For this review, take the finished solid that the model builds, in its own axes (mm). A direction names the side the tool comes from. Give positions to 0.01 mm unless a question says otherwise; leave off trailing zeros. Order: outer loops, then holes, each group sorted by start corner. A loop starts at its lowest first (then second) coordinate and runs counter-clockwise, first axis right, second up. Notation, with made-up numbers: M -20,75 L -15,75 A21 cw -15,106 Z; hole C -3,58 d6. An arc over 180 degrees is marked long. Use CSV: the item, a comma, the result in double quotes. Start each with the question number.
(1) Consider section C-C (z = -24.5). Write out the cut boundary in (x, y).
(2) Tool access review of faces 1 (the face through (51, 825, -4)), 2 (the face through (49, 828, 0)): name each direction out of +Z, -Z, +X, -X, +Y, -Y from which nothing blocks a thin tool from reaching the whole face with its end or side.
(3) Draft analysis for pull direction Z (two halves, no side actions). For faces 3 (the face through (97.915, 119.104, -46.063)), 4 (the face through (46, 1500, -2)), 5 (the face through (96, 771, -51)), state which applies: pulls with the +Z half, pulls with the -Z half, needs draft (parallel to the pull), parting line crosses it, or undercut.
(4) Wall thickness on L1, parallel to X at y = 1131, z = -84; L2, parallel to Z at x = 86, y = 979; L3, parallel to Z at x = 1, y = 1450: over which ranges is each line inside the solid? List them lowest first. Write a range as from..to.
(5) Clearance check with flat-ended pins moving along their axes: P1, Ø17.5, axis at y = 1450, z = -50, coming from the -X side; P2, Ø10, axis at x = 37.5, z = -13, coming from the +Y side. State where each tip first meets the part, or that it passes through.
(6) Consider section A-A (x = 80). Write out the cut boundary in (y, z), and give its area (3 significant figures).
(7) Consider section B-B (y = 1265.5). Write out the cut boundary in (x, z), and give its area (3 significant figures).
```python
from build123d import *

# Parameters (mm, degrees)
BOSS_EXTRU_1_DEPTH      = 1500
ESQUISSE4_R             = 6.75
ENL_V_MAT_EXTRU_1_DEPTH = 1507.651917332


with BuildPart() as part:
    # Esquisse2 → Boss.-Extru.1 (new body)
    with BuildSketch(Plane(origin=(0, 0, 0), x_dir=(1, 0, 0), z_dir=(0, 1, 0))):
        with BuildLine():
            Line((2, 0), (98, 0))
            ThreePointArc((98, 0), (99.414213562, 0.585786438), (100, 2))
            Line((100, 2), (100, 98))
            ThreePointArc((100, 98), (99.414213562, 99.414213562), (98, 100))
            Line((98, 100), (2, 100))
            ThreePointArc((2, 100), (0.585786438, 99.414213562), (0, 98))
            Line((0, 98), (0, 2))
            ThreePointArc((0, 2), (0.585786438, 0.585786438), (2, 0))
        make_face()
        with BuildLine():
            Line((6, 96), (94, 96))
            ThreePointArc((94, 96), (95.414213562, 95.414213562), (96, 94))
            Line((96, 94), (96, 6))
            ThreePointArc((96, 6), (95.414213562, 4.585786438), (94, 4))
            Line((94, 4), (6, 4))
            ThreePointArc((6, 4), (4.585786438, 4.585786438), (4, 6))
            Line((4, 6), (4, 94))
            ThreePointArc((4, 94), (4.585786438, 95.414213562), (6, 96))
        make_face(mode=Mode.SUBTRACT)
    extrude(amount=BOSS_EXTRU_1_DEPTH)

    # Esquisse4 → Enlèv. mat.-Extru.1 (cut, through all)
    with BuildSketch(Plane.ZY):
        with Locations((-50, 1450)):
            Circle(ESQUISSE4_R)
        with Locations((-50, 1098)):
            Circle(ESQUISSE4_R)
        Polygon((0, 174), (-165.464535812, -23.192955001), (56.265885145, -23.192955001), (56.265885145, 174), align=None)
    extrude(amount=-ENL_V_MAT_EXTRU_1_DEPTH, mode=Mode.SUBTRACT)


solid = part.part
```
Check result:
1,outline,"M 0,144.8 L 4,144.8 L 4,1500 L 0,1500 Z; M 96,144.8 L 100,144.8 L 100,1500 L 96,1500 Z"
2,face 1,"+Y, -Y"
2,face 2,"+Z, +X, -X, +Y, -Y"
3,face 3,"pulls with the +Z half"
3,face 4,"needs draft"
3,face 5,"undercut"
4,L1,"x = 0..4, 96..100"
4,L2,"z = -100..-96, -4..0"
4,L3,"z = -99.73..-56.75, -43.25..-0.27"
5,P1,"stops at x = 0"
5,P2,"passes through"
6,outline,"M 54.82,-100 L 1500,-100 L 1500,-96 L 59.59,-96 Z; M 169.23,-4 L 1500,-4 L 1500,0 L 174,0 Z"
6,area,"11,100 mm^2"
7,outline,"M 0,-98 A2 ccw 2,-100 L 98,-100 A2 ccw 100,-98 L 100,-2 A2 ccw 98,0 L 2,0 A2 ccw 0,-2 Z; hole M 4,-94 A2 ccw 6,-96 L 94,-96 A2 ccw 96,-94 L 96,-6 A2 ccw 94,-4 L 6,-4 A2 ccw 4,-6 Z"
7,area,"1,540 mm^2"
